The listing builds one solid part. Answer for the finished solid, in the listing's coordinates (mm). A direction names the side the tool comes from. Round coordinates to 2 decimals unless told otherwise and drop trailing zeros. Loops run counter-clockwise (first coordinate to the right, second up) from the corner with the lowest first, then second, coordinate; pieces in that order, holes last. Notation, with made-up numbers: M -22.5,-13 L -18.5,-13 A20 cw -18.5,-9 Z; hole C 26.25,20.25 d3. An arc over 180 degrees is marked long. Put each result on its own line as item: value. Start each with the question number.
(1) Section A-A, the plane z = -1.75 is taken. Determine the outline of the cut face in (x, y).
(2) Section B-B, the plane y = 1.3 is taken. Determine the outline of the cut face in (x, z).
(3) A flat-ended cylindrical pin translates along its axis: P1, Ø0.9, axis at y = 3.5, z = -2.5, coming from the +X side. Find the tip coordinate at first contact, or state that the pin passes through.
(4) Which of the six approach directions +Z, -Z, +X, -X, +Y, -Y give full straight-line access (tool end or side, diameter ignored) to faces 1 (the face through (-2, 2.9, -4)), 2 (the face through (-2, 1.5, -2.4)), 3 (the face through (202, 2.9, -4))?
(5) Straight lines are drawn through the part: line 1 (X direction, y = 3.5, z = -3.4); line 2 (X direction, y = 1.2, z = -3.75). For each, find the intervals that lie inside material, in ascending order.
```python
from build123d import *

# Parameters (mm, degrees)
ESQUISSE1_W        = 200
ESQUISSE1_H        = 5.5
BOSS_EXTRU_1_DEPTH = 4
CHANFREIN1_SIZE    = 0.4
BOSS_EXTRU_2_DEPTH = 2.9
CONG_1_R           = 0.4


with BuildPart() as part:
    # Esquisse1 → Boss.-Extru.1 (new body)
    with BuildSketch(Plane(origin=(0, 0, 0), x_dir=(1, 0, 0), z_dir=(0, 1, 0))):
        with Locations((100, 2.75)):
            Rectangle(ESQUISSE1_W, ESQUISSE1_H)
    extrude(amount=BOSS_EXTRU_1_DEPTH)

    # Chanfrein1
    chanfrein1_edges = [part.edges().sort_by_distance(p)[0] for p in [
        (200, 2, 0),
        (0, 2, 0),
    ]]
    chamfer(chanfrein1_edges, length=CHANFREIN1_SIZE)

    # Esquisse2 → Boss.-Extru.2 (add)
    with BuildSketch(Plane(origin=(0, 0, 0), x_dir=(1, 0, 0), z_dir=(0, 1, 0))):
        Polygon((0, 5.5), (-5.1, 5.5), (0, 0.4), align=None)
    boss_extru_2 = extrude(amount=BOSS_EXTRU_2_DEPTH)

    # Symétrie1: Boss.-Extru.2 across plane
    add(boss_extru_2.mirror(Plane.ZY.offset(-100)))

    # Congé1
    cong_1_edges = [part.edges().sort_by_distance(p)[0] for p in [
        (-5.1, 1.45, -5.5),
        (205.1, 1.45, -5.5),
    ]]
    fillet(cong_1_edges, radius=CONG_1_R)


solid = part.part
```
Recorded:
1. outline: M -1.35,0 L 201.35,0 L 201.35,2.9 L 200,2.9 L 200,4 L 0,4 L 0,2.9 L -1.35,2.9 Z
2. outline: M -4.42,-4.82 A0.4 ccw -4.13,-5.5 L 204.13,-5.5 A0.4 ccw 204.42,-4.82 L 199.6,0 L 0.4,0 Z
3. P1: stops at x = 200
4. face 1: +Z, -Z, -X, +Y
4. face 2: +Z, -X, +Y, -Y
4. face 3: +Z, -Z, +X, +Y
5. line 1: x = 0 to 200
5. line 2: x = -3.35 to 203.35
